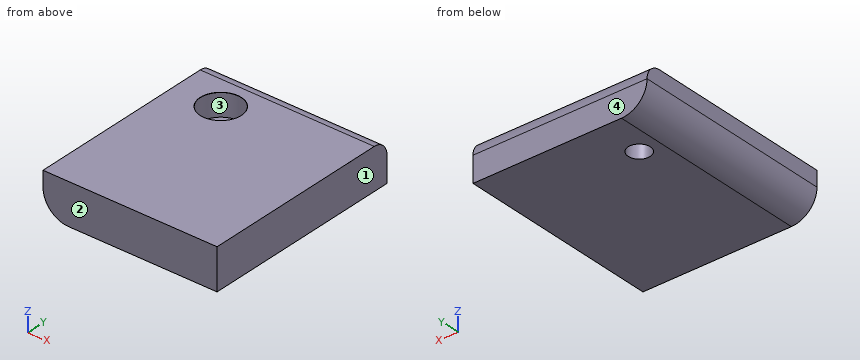
from build123d import *

# Parameters (mm, degrees)
SKETCH1_W                                    = 47
SKETCH1_H                                    = 8
BOSS_EXTRUDE1_DEPTH                          = 40
FILLET1_R                                    = 3
FILLET2_R                                    = 5
CBORE_FOR_M4_HEX_SOCKET_HEAD_CAP_SCR_2_COUNT = 2
CBORE_FOR_M4_HEX_SOCKET_HEAD_CAP_SCR_2_PITCH = 29
CUT_EXTRUDE1_REACH                           = 49.077
SKETCH5_W                                    = 13
SKETCH5_H                                    = 44.997787144


with BuildPart() as part:
    # Sketch1 → Boss-Extrude1 (new body)
    with BuildSketch(Plane(origin=(0, 0, 0), x_dir=(1, 0, 0), z_dir=(0, 1, 0))):
        Rectangle(SKETCH1_W, SKETCH1_H)
    extrude(amount=-BOSS_EXTRUDE1_DEPTH)

    # Fillet1
    fillet1_edges = [part.edges().sort_by_distance(p)[0] for p in [
        (0, 0, 4),
    ]]
    fillet(fillet1_edges, radius=FILLET1_R)

    # Fillet2
    fillet2_edges = [part.edges().sort_by_distance(p)[0] for p in [
        (-23.5, -20, -4),
        (23.5, -20, -4),
    ]]
    fillet(fillet2_edges, radius=FILLET2_R)

    # Sketch3 → CBORE for M4 Hex Socket Head Cap Screw1 (revolve, cut)
    with BuildSketch(Plane(origin=(-14.5, -9, 4), x_dir=(0, -1, 0), z_dir=(1, 0, 0))):
        Polygon((0, 0), (0, 8), (2.15, 8), (2.15, 4.4), (4, 4.4), (4, 0.025), (4.025, 0), align=None)
    cbore_for_m4_hex_socket_head_cap_screw1 = revolve(axis=Axis((-14.5, -9, 10.35), (0, 0, -1)), mode=Mode.SUBTRACT)

    # CBORE for M4 Hex Socket Head Cap Scr 2: CBORE for M4 Hex Socket Head Cap Screw1 ×2
    with Locations(*[(i * CBORE_FOR_M4_HEX_SOCKET_HEAD_CAP_SCR_2_PITCH, 0, 0) for i in range(1, CBORE_FOR_M4_HEX_SOCKET_HEAD_CAP_SCR_2_COUNT)]):
        add(cbore_for_m4_hex_socket_head_cap_screw1, mode=Mode.SUBTRACT)

    # Sketch5 → Cut-Extrude1 (cut, up to next)
    with BuildSketch(Plane.XY.offset(4), mode=Mode.PRIVATE) as cut_extrude1_sk1:
        with Locations((17, -17.501106428)):
            Rectangle(SKETCH5_W, SKETCH5_H)
    cut_extrude1_tool1 = extrude(cut_extrude1_sk1.sketch, amount=-CUT_EXTRUDE1_REACH, mode=Mode.PRIVATE) & part.part
    add(cut_extrude1_tool1.solids().sort_by_distance((17, -17.501106, 4))[0], mode=Mode.SUBTRACT)


solid = part.part
Read the model definition and answer for the solid it produces. Units are mm, in the model's axes. Face numbers are marked on the shaded views. Round coordinates to 2 decimals unless told otherwise and drop trailing zeros. Write each loop counter-clockwise with the first axis right and the second up, starting at its lowest first coordinate (ties: lowest second). Pieces come first, ordered by that corner, then holes. Notation, with made-up numbers: (-20, 78) - (36, 78) arc R26 cw to (36, 102) - close; hole circle Ø8 at (45.5, 24.25). An arc over 180 degrees is marked (long way). Use a Markdown table: item, result.
(1) The part is cut by section A-A (y = -9). Write down the section's boundary in (x, z) (3 decimals), then the cut area to 3 significant figures.
Reported:
| item | result |
|---|---|
| outline | (-23.5, 1) arc R5 ccw to (-18.5, -4) - (-16.65, -4) - (-16.65, -0.4) - (-18.5, -0.4) - (-18.5, 3.975) - (-18.525, 4) - (-23.5, 4) - close; (-12.35, -4) - (10.5, -4) - (10.5, 3.975) - (10.475, 4) - (-10.475, 4) - (-10.5, 3.975) - (-10.5, -0.4) - (-12.35, -0.4) - close |
| area | 216 mm2 |
(2) The mould has two halves that part along Y. Classify the marked faces 1, 2, 3 and 4: released by +Y, released by -Y, zero draft, split by the parting line, or undercut.
Reported:
| item | result |
|---|---|
| face 1 | zero draft |
| face 2 | released by -Y |
| face 3 | undercut |
| face 4 | released by +Y |
(3) Straight lines are drawn through the part: line 1 along Y through (x, z) = (-14.5, -2.65); line 2 along X through (y, z) = (-9, 3.1); line 3 along Y through (x, z) = (-15, 2.5). For each, find the intervals that lie inside material, in ascending order. Write a range as [from, to].
Reported:
| item | result |
|---|---|
| line 1 | [-40, -11.15], [-6.85, 0] |
| line 2 | [-23.5, -18.5], [-10.5, 10.5] |
| line 3 | [-40, -12.97], [-5.03, -0.4] |
(4) The part is cut by section C-C (y = -21.5). Write down the section's boundary in (x, z), then the cut area to 3 significant figures.
Reported:
| item | result |
|---|---|
| outline | (-23.5, 1) arc R5 ccw to (-18.5, -4) - (10.5, -4) - (10.5, 4) - (-23.5, 4) - close |
| area | 267 mm2 |
(5) Each of these flat-tipped pins is pushed along its axis until it touches: pin 1 Ø3 at (y, z) = (-25.5, -1.5) entering from -X; pin 2 Ø3 at (y, z) = (-14.5, -3) entering from -X. Where does it stop, or does it pass through?
Reported:
| item | result |
|---|---|
| pin 1 | x = -23.4 |
| pin 2 | x = -22.83 |
(6) The part is cut by section B-B (x = -14.5). Write down the section's boundary in (y, z) (3 decimals), then the cut area to 3 significant figures.
Reported:
| item | result |
|---|---|
| outline | (-40, -4) - (-11.15, -4) - (-11.15, -0.4) - (-13, -0.4) - (-13, 3.975) - (-13.025, 4) - (-40, 4) - close; (-6.85, -4) - (0, -4) - (0, 1) arc R3 ccw to (-3, 4) - (-4.975, 4) - (-5, 3.975) - (-5, -0.4) - (-6.85, -0.4) - close |
| area | 267 mm2 |
(7) The part is cut by section D-D (z = -1.25). Write down the section's boundary in (x, y).
Reported:
| item | result |
|---|---|
| outline | (-22.97, -40) - (10.5, -40) - (10.5, 0) - (-22.97, 0) - close; hole circle Ø4.3 at (-14.5, -9) |
